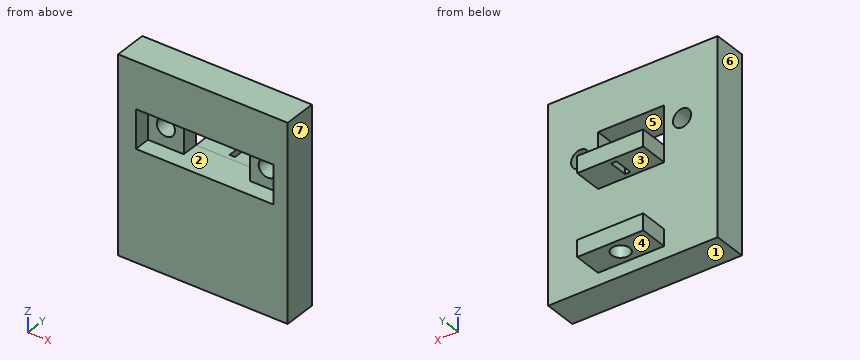
from build123d import *

# Parameters (mm, degrees)
F0_W     = 30.7991821319
F0_H     = 35.4098370299
F0_W_2   = 6.5
F0_H_2   = 7
F1_DEPTH = 6
F2_DEPTH = 3
F3_D     = 3.3
F4_W     = 12
F4_H     = 3
F5_DEPTH = 5.2
F6_W     = 0.9753258782
F6_H     = 3.4873990223
F7_DEPTH = 3
F9_D     = 3.3
F9_DEPTH = 5.2341906781


with BuildPart() as f1:
    # F0 (on Front) → F1 (new body)
    with BuildSketch(Plane.XZ):
        with Locations((-0.321273692, 7.8438320197)):
            Rectangle(F0_W, F0_H)
        Polygon((-12.4934045598, 17.1573571861), (-5.9934045598, 17.1573571861), (6.0065954402, 17.1573571861), (12.5065954402, 17.1573571861), (12.5065954402, 10.1573571861), (6.0065954402, 10.1573571861), (-5.9934045598, 10.1573571861), (-12.4934045598, 10.1573571861), align=None, mode=Mode.SUBTRACT)
        with Locations((-9.2434045598, 13.6573571861)):
            Rectangle(F0_W_2, F0_H_2)
        with Locations((9.2565954402, 13.6573571861)):
            Rectangle(F0_W_2, F0_H_2)
    extrude(amount=-F1_DEPTH)

    # F0 (on Front) → F2 (cut)
    with BuildSketch(Plane.XZ):
        with Locations((-9.2434045598, 13.6573571861)):
            Rectangle(F0_W_2, F0_H_2)
        with Locations((9.2565954402, 13.6573571861)):
            Rectangle(F0_W_2, F0_H_2)
    extrude(amount=-F2_DEPTH, mode=Mode.SUBTRACT)

    # F3 (through all)
    with Locations(Plane.XZ):
        with Locations((-9.2434045598, 13.6573571861), (9.2565954402, 13.6573571861)):
            Hole(F3_D / 2)

    # F4 (on face) → F5 (join)
    with BuildSketch(Plane(origin=(0, 6, 0), x_dir=(-1, 0, 0), z_dir=(0, 1, 0))):
        with Locations((-0.0065954402, -6.1278958172)):
            Rectangle(F4_W, F4_H)
        with Locations((-0.0065954402, 8.6368762217)):
            Rectangle(F4_W, F4_H)
    extrude(amount=F5_DEPTH)

    # F6 (on face) → F7 (cut, through all)
    with BuildSketch(Plane.XY.offset(10.1368762217)):
        with Locations((0, 8.5971419759)):
            Rectangle(F6_W, F6_H)
    extrude(amount=-F7_DEPTH, mode=Mode.SUBTRACT)

    # F9 (through all, one way)
    with BuildSketch(Plane.XY.offset(-4.6278958172)):
        with Locations((0.0065954402, 8.6)):
            Circle(F9_D / 2)
    extrude(amount=-F9_DEPTH, mode=Mode.SUBTRACT)


solid = f1.part
For this review, take the finished solid that the model builds, in its own axes (mm). Face numbers are marked on the shaded views. A direction names the side the tool comes from. Give positions to 0.01 mm unless a question says otherwise; leave off trailing zeros. Loops run counter-clockwise (first coordinate to the right, second up) from the corner with the lowest first, then second, coordinate; pieces in that order, holes last. Notation, with made-up numbers: M 46,-32 L 86,-32 A28 cw 86,-3 Z; hole C 53.25,0.5 d11. An arc over 180 degrees is marked long. Answer as a JSON object with one key per item and string values. Group by question number.
Q1. Insertion check: P1, Ø2.5, axis at x = -9.24, z = 13.66, coming from the -Y side; P2, Ø2, axis at x = 0.01, y = 8.6, coming from the -Z side; P3, Ø1.6, axis at x = -1, y = 8, coming from the -Z side; P4, Ø3.5, axis at y = 9.5, z = 9.5, coming from the +X side. Each pin has a flat end and moves straight along its axis. Give the tip position at first contact, or say it passes through.
Q2. Add section B-B on y = 1.5. Give the boundary of the cut face in (x, z).
Q3. Add section D-D on y = 3.5. Give the boundary of the cut face in (x, z).
Q4. Tool access review of the marked faces 1, 2 and 3: name each direction out of +Z, -Z, +X, -X, +Y, -Y from which nothing blocks a thin tool from reaching the whole face with its end or side.
Q5. Add section C-C on z = 6.5. Give the boundary of the cut face in (x, y).
Q6. Add section A-A on y = 8.6. Give the boundary of the cut face in (x, z), and give its area (3 significant figures).
Q7. For probe 1 along X at (y, z) = (5, 11); probe 2 along Z at (x, y) = (5, 8.5); probe 3 along X at (y, z) = (2, 11), list the stretches that pass through material, from the lowest coordinate up. Write a range as [from, to].
Q8. Mouldability with a two-part tool opening along X and no side actions: class the marked faces 4, 5, 6 and 7 as +X half, -X half, draft (parallel to the pull), parting line (faces both ways), or undercut.
Checked values:
{
 "1": {"P1": "through", "P2": "z = 7.14", "P3": "z = -7.63", "P4": "x = 6.01"},
 "2": {"outline": "M -15.72,-9.86 L 15.08,-9.86 L 15.08,25.55 L -15.72,25.55 Z; hole M -12.49,10.16 L 12.51,10.16 L 12.51,17.16 L -12.49,17.16 Z"},
 "3": {"outline": "M -15.72,-9.86 L 15.08,-9.86 L 15.08,25.55 L -15.72,25.55 Z; hole C -9.24,13.66 d3.3; hole M -5.99,10.16 L 6.01,10.16 L 6.01,17.16 L -5.99,17.16 Z; hole C 9.26,13.66 d3.3"},
 "4": {"face 1": "-Z, +X, -X, +Y, -Y", "face 2": "-Y", "face 3": "+X, -X, +Y"},
 "5": {"outline": "M -15.72,0 L 15.08,0 L 15.08,6 L -15.72,6 Z"},
 "6": {"outline": "M -5.99,-7.63 L -1.64,-7.63 L -1.64,-4.63 L -5.99,-4.63 Z; M -5.99,7.14 L -0.49,7.14 L -0.49,10.14 L -5.99,10.14 Z; M 0.49,7.14 L 6.01,7.14 L 6.01,10.14 L 0.49,10.14 Z; M 1.66,-7.63 L 6.01,-7.63 L 6.01,-4.63 L 1.66,-4.63 Z", "area": "59.2 mm²"},
 "7": {"probe 1": "[-15.72, -5.99], [6.01, 15.08]", "probe 2": "[-7.63, -4.63], [7.14, 10.14]", "probe 3": "[-15.72, -12.49], [12.51, 15.08]"},
 "8": {"face 4": "draft", "face 5": "undercut", "face 6": "-X half", "face 7": "+X half"}
}
